```python
from build123d import *

# Parameters (mm, degrees)
BASE_EXTRUDE_DEPTH = 3


with BuildPart() as part:
    # Sketch1 → Base-Extrude (new body)
    with BuildSketch(Plane.XY):
        with BuildLine():
            Line((693.938729313, -90.783662266), (693.938729313, -115.783662266))
            Line((693.938729313, -115.783662266), (687.938729313, -115.783662266))
            Line((687.938729313, -115.783662266), (687.938729313, -118.783662266))
            Line((687.938729313, -118.783662266), (693.938729313, -118.783662266))
            Line((693.938729313, -118.783662266), (693.938729313, -121.233634181))
            Line((693.938729313, -121.233634181), (687.938729313, -121.233634181))
            Line((687.938729313, -121.233634181), (687.938729313, -124.233634181))
            Line((687.938729313, -124.233634181), (693.938729313, -124.233634181))
            Line((693.938729313, -124.233634181), (693.938729313, -129.532471762))
            ThreePointArc((693.938729313, -129.532471762), (685.843524958, -130.127844479), (677.938729313, -128.283662266))
            Line((677.938729313, -128.283662266), (677.938729313, -111.479521793))
            Line((677.938729313, -111.479521793), (683.467463006, -111.479521793))
            Line((683.467463006, -111.479521793), (683.467463006, -108.479521793))
            Line((683.467463006, -108.479521793), (677.938729313, -108.479521793))
            Line((677.938729313, -108.479521793), (677.938729313, -98.087802738))
            Line((677.938729313, -98.087802738), (683.467463006, -98.087802738))
            Line((683.467463006, -98.087802738), (683.467463006, -95.087802738))
            Line((683.467463006, -95.087802738), (677.938729313, -95.087802738))
            Line((677.938729313, -95.087802738), (677.938729313, -78.283662266))
            ThreePointArc((677.938729313, -78.283662266), (685.843524958, -76.439480052), (693.938729313, -77.034852769))
            Line((693.938729313, -77.034852769), (693.938729313, -82.33369035))
            Line((693.938729313, -82.33369035), (687.938729313, -82.33369035))
            Line((687.938729313, -82.33369035), (687.938729313, -85.33369035))
            Line((687.938729313, -85.33369035), (693.938729313, -85.33369035))
            Line((693.938729313, -85.33369035), (693.938729313, -87.783662266))
            Line((693.938729313, -87.783662266), (687.938729313, -87.783662266))
            Line((687.938729313, -87.783662266), (687.938729313, -90.783662266))
            Line((687.938729313, -90.783662266), (693.938729313, -90.783662266))
        make_face()
    extrude(amount=BASE_EXTRUDE_DEPTH)


solid = part.part
```
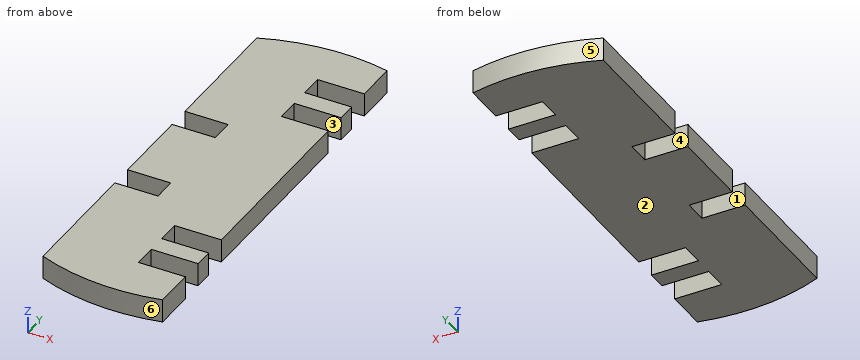
Source: CAD feature listing. Evaluate the final solid. Frame: model axes, mm. Face numbers are marked on the shaded views. A direction names the side the tool comes from. Give positions to 0.01 mm unless a question says otherwise; leave off trailing zeros. Write each loop counter-clockwise with the first axis right and the second up, starting at its lowest first coordinate (ties: lowest second). Pieces come first, ordered by that corner, then holes. Notation, with made-up numbers: (-17, 65.25) - (6, 65.25) arc R4 ccw to (6, 71.25) - close; hole circle Ø9 at (-2.5, 72.25). An arc over 180 degrees is marked (long way). One line per item, written item: value. Start each with the question number.
Q1. Section query D-D, the plane y = -89. Return the cut outline in (x, z).
Q2. Draft query along Y for the marked faces 4, 5 and 6. Return one class per face: +Y half, -Y half, draft (parallel to the pull), parting line (faces both ways), or undercut.
Q3. Section query B-B, the plane z = 0.9. Return the cut outline in (x, y).
Q4. Set-up query: the marked faces 1, 2 and 3. Return all of +Z, -Z, +X, -X, +Y, -Y with unobstructed straight access to the full face (end or side cutting, diameter ignored); none if empty.
Q5. Section query A-A, the plane x = 690.25. Return the cut outline in (y, z), then the cut area to 3 significant figures.
Q6. Section query C-C, the plane x = 680. Return the cut outline in (y, z).
Q7. Material intervals for probe 1 along Y at (x, z) = (688.5, 1.9); probe 2 along Y at (x, z) = (690.25, 2.8); probe 3 along Y at (x, z) = (682.25, 2.3), sorted ascending. Write a range as from..to.
Q8. First-contact query: pin 1 Ø0.9 at (y, z) = (-110.5, 1.5) entering from -X; pin 2 Ø1.5 at (y, z) = (-121.5, 1) entering from +X; pin 3 Ø1.5 at (x, z) = (681.5, 1.5) entering from -Y; pin 4 Ø1.5 at (x, z) = (691.5, 2) entering from -Y. Flat tips, straight axial feed; report the tip coordinate or a pass-through.
Answer:
1. outline: (677.94, 0) - (687.94, 0) - (687.94, 3) - (677.94, 3) - close
2. face 4: undercut
2. face 5: +Y half
2. face 6: -Y half
3. outline: (677.94, -128.28) arc R26.93 ccw to (693.94, -129.53) - (693.94, -124.23) - (687.94, -124.23) - (687.94, -121.23) - (693.94, -121.23) - (693.94, -118.78) - (687.94, -118.78) - (687.94, -115.78) - (693.94, -115.78) - (693.94, -90.78) - (687.94, -90.78) - (687.94, -87.78) - (693.94, -87.78) - (693.94, -85.33) - (687.94, -85.33) - (687.94, -82.33) - (693.94, -82.33) - (693.94, -77.03) arc R26.93 ccw to (677.94, -78.28) - (677.94, -95.09) - (683.47, -95.09) - (683.47, -98.09) - (677.94, -98.09) - (677.94, -108.48) - (683.47, -108.48) - (683.47, -111.48) - (677.94, -111.48) - close
4. face 1: +Z, -Z, -X
4. face 2: -Z, +X, -X, +Y, -Y
4. face 3: +Z, -Z, +X
5. outline: (-130.11, 0) - (-124.23, 0) - (-124.23, 3) - (-130.11, 3) - close; (-121.23, 0) - (-118.78, 0) - (-118.78, 3) - (-121.23, 3) - close; (-115.78, 0) - (-90.78, 0) - (-90.78, 3) - (-115.78, 3) - close; (-87.78, 0) - (-85.33, 0) - (-85.33, 3) - (-87.78, 3) - close; (-82.33, 0) - (-76.46, 0) - (-76.46, 3) - (-82.33, 3) - close
5. area: 125 mm2
6. outline: (-129.01, 0) - (-111.48, 0) - (-111.48, 3) - (-129.01, 3) - close; (-108.48, 0) - (-98.09, 0) - (-98.09, 3) - (-108.48, 3) - close; (-95.09, 0) - (-77.55, 0) - (-77.55, 3) - (-95.09, 3) - close
7. probe 1: y = -130.2..-124.23, -121.23..-118.78, -115.78..-90.78, -87.78..-85.33, -82.33..-76.36
7. probe 2: y = -130.11..-124.23, -121.23..-118.78, -115.78..-90.78, -87.78..-85.33, -82.33..-76.46
7. probe 3: y = -129.6..-111.48, -108.48..-98.09, -95.09..-76.97
8. pin 1: stops at x = 683.47
8. pin 2: stops at x = 693.94
8. pin 3: stops at y = -129.6
8. pin 4: stops at y = -130.06
